```python
from build123d import *

# Parameters (mm, degrees)
SKETCH1_W               = 40.386
SKETCH1_H               = 40.132
BOSS_EXTRUDE1_DEPTH     = 19.05
SKETCH2_W               = 7.239
SKETCH2_H               = 3.048
BOSS_EXTRUDE2_DEPTH     = 19.05
SKETCH3_R               = 2.54
CUT_EXTRUDE1_DEPTH      = 11.16
CUT_EXTRUDE1_DEPTH_BACK = 30.972
SKETCH4_R               = 3.81
BOSS_EXTRUDE3_DEPTH     = 5.588
SKETCH5_W               = 9.05
SKETCH5_H               = 4
BOSS_EXTRUDE4_DEPTH     = 6
BOSS_EXTRUDE5_DEPTH     = 1


with BuildPart() as part:
    # Sketch1 → Boss-Extrude1 (new body)
    with BuildSketch(Plane.XY):
        with Locations((20.193, 20.066)):
            Rectangle(SKETCH1_W, SKETCH1_H)
    extrude(amount=BOSS_EXTRUDE1_DEPTH)

    # Sketch2 → Boss-Extrude2 (add)
    with BuildSketch(Plane.XY.offset(19.05)):
        with Locations((-3.6195, 28.448)):
            Rectangle(SKETCH2_W, SKETCH2_H)
        with Locations((44.0055, 28.448)):
            Rectangle(SKETCH2_W, SKETCH2_H)
    extrude(amount=-BOSS_EXTRUDE2_DEPTH)

    # Sketch3 → Cut-Extrude1 (cut, two sides)
    with BuildSketch(Plane(origin=(0, 29.972, 0), x_dir=(1, 0, 0), z_dir=(0, 1, 0))) as cut_extrude1_sk:
        with Locations((-3.937, -14.351)):
            Circle(SKETCH3_R)
        with Locations((-3.937, -4.699)):
            Circle(SKETCH3_R)
        with Locations((44.323, -14.351)):
            Circle(SKETCH3_R)
        with Locations((44.323, -4.699)):
            Circle(SKETCH3_R)
    extrude(amount=CUT_EXTRUDE1_DEPTH, mode=Mode.SUBTRACT)
    extrude(cut_extrude1_sk.sketch, amount=-CUT_EXTRUDE1_DEPTH_BACK, mode=Mode.SUBTRACT)

    # Sketch4 → Boss-Extrude3 (add)
    with BuildSketch(Plane(origin=(0, 40.132, 0), x_dir=(1, 0, 0), z_dir=(0, 1, 0))):
        with Locations((9.66, -9.525)):
            Circle(SKETCH4_R)
    extrude(amount=BOSS_EXTRUDE3_DEPTH)

    # Sketch5 → Boss-Extrude4 (add)
    with BuildSketch(Plane.ZY):
        with Locations((9.525, 5.048)):
            Rectangle(SKETCH5_W, SKETCH5_H)
    extrude(amount=BOSS_EXTRUDE4_DEPTH)

    # Sketch7 → Boss-Extrude5 (add, symmetric)
    with BuildSketch(Plane.XY.offset(9.525)):
        Polygon((-6.35, 29.972), (0, 32.512), (0, 29.972), align=None)
        Polygon((45.466, 29.972), (40.386, 34.55105012), (40.386, 29.972), align=None)
    extrude(amount=BOSS_EXTRUDE5_DEPTH, both=True)


solid = part.part
```
The model under review builds one solid part; all positions refer to its coordinate system, in mm. A direction names the side the tool comes from. Round coordinates to 2 decimals unless told otherwise and drop trailing zeros. Loops run counter-clockwise (first coordinate to the right, second up) from the corner with the lowest first, then second, coordinate; pieces in that order, holes last. Notation, with made-up numbers: (69, 6.5) - (82, 6.5) arc R24 cw to (82, 35.5) - close; hole circle Ø6 at (-12, -30). An arc over 180 degrees is marked (long way). Write each question's results on one line, items separated by ' | '. Start each with the question number.
Q1. Take a section at C-C on y = 4.5. Give the boundary of the cut face in (x, z), plus the area to 3 significant figures.
Q2. Take a section at B-B on y = 28. Give the boundary of the cut face in (x, z) (3 decimals), plus the area to 3 significant figures.
Q3. Take a section at A-A on x = 9.66. Give the boundary of the cut face in (y, z) (3 decimals).
Q4. Tool access review of faces 1 (the flat face through (-2, 31, 8.525)), 2 (the cylindrical face through (-4.268, 28.469, 11.833)), 3 (the flat face through (42, 31, 10.525)), 4 (the flat face through (40.386, 13, 9)), 5 (the flat face through (-3, 3.048, 9)): name each direction out of +Z, -Z, +X, -X, +Y, -Y from which nothing blocks a thin tool from reaching the whole face with its end or side.
Q5. Wall thickness on line 1 along Y through (x, z) = (19.5, 7.25); line 2 along X through (y, z) = (2, 14); line 3 along Y through (x, z) = (-1, 8.25): over which ranges is each line inside the solid? List them lowest first. Write a range as [from, to].
Q6. Take a section at D-D on x = 16.5. Give the boundary of the cut face in (y, z).
Q7. Insertion check: P1, Ø3, axis at y = 32.5, z = 7.5, coming from the +X side; P2, Ø9.5, axis at x = 29, z = 7, coming from the +Y side; P3, Ø2, axis at x = -2.5, y = 31.5, coming from the -Z side (3 decimals). Each pin has a flat end and moves straight along its axis. Give the tip position at first contact, or say it passes through.
Q8. Draft analysis for pull direction Z (two halves, no side actions). For faces 6 (the flat face through (20, 20, 19.05)), 7 (the flat face through (44, 26.924, 10)), 8 (the cylindrical face through (46.746, 28.469, 13.588)), state which applies: pulls with the +Z half, pulls with the -Z half, needs draft (parallel to the pull), parting line crosses it, or undercut.
Data:
1) outline: (-6, 5) - (0, 5) - (0, 0) - (40.39, 0) - (40.39, 19.05) - (0, 19.05) - (0, 14.05) - (-6, 14.05) - close | area: 824 mm²
2) outline: (-7.239, 0) - (47.625, 0) - (47.625, 19.05) - (-7.239, 19.05) - close; hole circle Ø5.08 at (-3.937, 4.699); hole circle Ø5.08 at (-3.937, 14.351); hole circle Ø5.08 at (44.323, 4.699); hole circle Ø5.08 at (44.323, 14.351) | area: 964 mm²
3) outline: (0, 0) - (40.132, 0) - (40.132, 5.715) - (45.72, 5.715) - (45.72, 13.335) - (40.132, 13.335) - (40.132, 19.05) - (0, 19.05) - close
4) face 1: -Z, -X, +Y | face 2: +Y | face 3: +Z, +X, +Y | face 4: +Z, -Z, +X, -Y | face 5: +Z, -Z, -X, -Y
5) line 1: y = [0, 40.13] | line 2: x = [0, 40.39] | line 3: y = [3.05, 7.05], [26.92, 29.97]
6) outline: (0, 0) - (40.13, 0) - (40.13, 19.05) - (0, 19.05) - close
7) P1: stops at x = 43.88 | P2: stops at y = 40.13 | P3: stops at z = 8.525
8) face 6: pulls with the +Z half | face 7: needs draft | face 8: undercut
